CAD build for the part. Positions are in the model's coordinates, mm. Face numbers are marked on the shaded views. Round coordinates to 2 decimals unless told otherwise and drop trailing zeros. Loops run counter-clockwise (first coordinate to the right, second up) from the corner with the lowest first, then second, coordinate; pieces in that order, holes last.
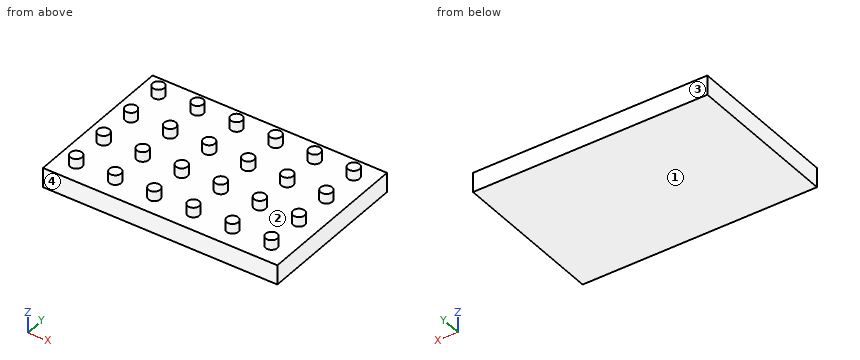
Autodesk Inventor part; units mm, degrees
ref_plane "YZ Plane" through (0, 0, 0) normal (1, 0, 0) x (0, 1, 0)
ref_plane "XZ Plane" through (0, 0, 0) normal (0, 1, 0) x (-1, 0, 0)
ref_plane "XY Plane" through (0, 0, 0) normal (0, 0, 1) x (1, 0, 0)
sketch "Sketch1" plane through (0, 0, 0) normal (0, 0, 1) x (1, 0, 0)
  line L0 (0, 0) -> (152.4, 0)
  line L1 (152.4, 0) -> (152.4, 101.6)
  line L2 (152.4, 101.6) -> (0, 101.6)
  line L3 (0, 101.6) -> (0, 0)
  dimension "d0" = 152.4
  dimension "d1" = 101.6
extrude "Extrusion1" add sketch "Sketch1" along normal blind 12.7
sketch "Sketch2" plane through (0, 0, 12.7) normal (0, 0, 1) x (1, 0, 0)
  circle A0 centre (12.7, 12.7) radius 3.81
  line L0 (0, 101.6) -> (0, 0)
  line L1 (0, 0) -> (152.4, 0)
  dimension "d4" = 12.7
  dimension "d5" = 12.7
  dimension "d6" = 7.62
extrude "Extrusion2" add sketch "Sketch2" along normal blind 6.35
pattern_linear "Rectangular Pattern1" count 6 spacing 25.4 along (1, 0, 0) count 4 spacing 25.4 along (0, 1, 0) of "Extrusion2"
properties part number "Rectangle Pattern Practice"
Item 1: Mould opens along Y. For the marked faces 1, 2, 3 and 4 say: released by +Y, released by -Y, zero draft, split by the parting line, or undercut.
Verdict:
face 1: zero draft
face 2: undercut
face 3: released by +Y
face 4: released by -Y
Item 2: Cut at C-C (x = 139.7). List the corners of the cut face in (y, z).
Verdict:
outline: (0, 0) - (101.6, 0) - (101.6, 12.7) - (92.71, 12.7) - (92.71, 19.05) - (85.09, 19.05) - (85.09, 12.7) - (67.31, 12.7) - (67.31, 19.05) - (59.69, 19.05) - (59.69, 12.7) - (41.91, 12.7) - (41.91, 19.05) - (34.29, 19.05) - (34.29, 12.7) - (16.51, 12.7) - (16.51, 19.05) - (8.89, 19.05) - (8.89, 12.7) - (0, 12.7) - close
Item 3: Flat gauge pin, fed straight in: P1, Ø12, axis at x = 85, y = 27, coming from the +Z side. Where does the tip first touch, or does it go through?
Verdict:
P1: stops at z = 12.7
Item 4: Wall check: L1, parallel to Y at x = 112.5, z = 17.75; L2, parallel to Y at x = 117.5, z = 14.5; L3, parallel to Z at x = 96.5, y = 89.5. Give the ranges that are in metal, low to high.
Verdict:
L1: y = 9.34 to 16.06, 34.74 to 41.46, 60.14 to 66.86, 85.54 to 92.26
L2: y = 10.63 to 14.77, 36.03 to 40.17, 61.43 to 65.57, 86.83 to 90.97
L3: z = 0 to 12.7
Item 5: Cut at B-B (y = 63.5). List the corners of the cut face in (x, z), plus the area to 3 significant figures.
Verdict:
outline: (0, 0) - (152.4, 0) - (152.4, 12.7) - (143.51, 12.7) - (143.51, 19.05) - (135.89, 19.05) - (135.89, 12.7) - (118.11, 12.7) - (118.11, 19.05) - (110.49, 19.05) - (110.49, 12.7) - (92.71, 12.7) - (92.71, 19.05) - (85.09, 19.05) - (85.09, 12.7) - (67.31, 12.7) - (67.31, 19.05) - (59.69, 19.05) - (59.69, 12.7) - (41.91, 12.7) - (41.91, 19.05) - (34.29, 19.05) - (34.29, 12.7) - (16.51, 12.7) - (16.51, 19.05) - (8.89, 19.05) - (8.89, 12.7) - (0, 12.7) - close
area: 2,230 mm2
Item 6: Cut at A-A (z = 15.75). State how many separate pieces and enclosed holes the cut face has, plus the area to 3 significant figures.
Verdict:
separate pieces: 24
enclosed holes: 0
area: 1,090 mm2
Item 7: Cut at D-D (x = 50.5). List the corners of the cut face in (y, z), plus the area to 3 significant figures.
Verdict:
outline: (0, 0) - (101.6, 0) - (101.6, 12.7) - (0, 12.7) - close
area: 1,290 mm2
